Geometry: final body of the model. Coordinates: model frame, mm. A direction names the side the tool comes from. Round coordinates to 2 decimals unless told otherwise and drop trailing zeros. Write each loop counter-clockwise with the first axis right and the second up, starting at its lowest first coordinate (ties: lowest second). Pieces come first, ordered by that corner, then holes. Notation, with made-up numbers: (52.5, 58) -> (86.5, 58) arc R12 ccw to (86.5, 73) -> close; hole circle Ø9 at (70, 65.5). An arc over 180 degrees is marked (long way). One line per item, written item: value. Start each with the question number.
from build123d import *

# Parameters (mm, degrees)
AUFSATZ_LINEAR_AUSTRAGEN1_DEPTH = 120
SCHNITT_LINEAR_AUSTRAGEN1_DEPTH = 10
SKIZZE3_R                       = 3
SKIZZE3_R_2                     = 3.5
SCHNITT_LINEAR_AUSTRAGEN2_DEPTH = 60


with BuildPart() as part:
    # Skizze1 → Aufsatz-Linear austragen1 (new body)
    with BuildSketch(Plane.XY):
        with BuildLine():
            Line((0, 35), (0, 5))
            ThreePointArc((0, 5), (1.464466094, 1.464466094), (5, 0))
            Line((5, 0), (75, 0))
            ThreePointArc((75, 0), (78.535533906, 1.464466094), (80, 5))
            Line((80, 5), (80, 35))
            ThreePointArc((80, 35), (78.535533906, 38.535533906), (75, 40))
            Line((75, 40), (5, 40))
            ThreePointArc((5, 40), (1.464466094, 38.535533906), (0, 35))
        make_face()
        with BuildLine():
            Line((78, 5), (78, 35))
            ThreePointArc((78, 35), (77.121320344, 37.121320344), (75, 38))
            Line((75, 38), (5, 38))
            ThreePointArc((5, 38), (2.878679656, 37.121320344), (2, 35))
            Line((2, 35), (2, 5))
            ThreePointArc((2, 5), (2.878679656, 2.878679656), (5, 2))
            Line((5, 2), (75, 2))
            ThreePointArc((75, 2), (77.121320344, 2.878679656), (78, 5))
        make_face(mode=Mode.SUBTRACT)
    extrude(amount=AUFSATZ_LINEAR_AUSTRAGEN1_DEPTH)

    # Skizze2 → Schnitt-Linear austragen1 (cut)
    with BuildSketch(Plane.XZ):
        with BuildLine():
            Line((9, 120), (71, 120))
            Line((71, 120), (71, 75))
            ThreePointArc((71, 75), (69.535533906, 71.464466094), (66, 70))
            Line((66, 70), (14, 70))
            ThreePointArc((14, 70), (10.464466094, 71.464466094), (9, 75))
            Line((9, 75), (9, 120))
        make_face()
    extrude(amount=-SCHNITT_LINEAR_AUSTRAGEN1_DEPTH, mode=Mode.SUBTRACT)

    # Skizze3 → Schnitt-Linear austragen2 (cut)
    with BuildSketch(Plane(origin=(0, 40, 0), x_dir=(1, 0, 0), z_dir=(0, 1, 0))):
        with Locations(Location((60, -20, 0), (0, 0, 180))):
            Circle(SKIZZE3_R)
        with Locations(Location((20, -20, 0), (0, 0, 180))):
            Circle(SKIZZE3_R)
        with Locations(Location((60, -60, 0), (0, 0, 180))):
            Circle(SKIZZE3_R)
        with Locations(Location((20, -60, 0), (0, 0, 180))):
            Circle(SKIZZE3_R)
        with Locations(Location((63, -107, 0), (0, 0, 180))):
            Circle(SKIZZE3_R_2)
        with Locations(Location((17, -107, 0), (0, 0, 180))):
            Circle(SKIZZE3_R_2)
    extrude(amount=-SCHNITT_LINEAR_AUSTRAGEN2_DEPTH, mode=Mode.SUBTRACT)


solid = part.part
(1) Pull-direction query (Z, two-part tool) for faces 3 (the face through (11, 1, 71)), 4 (the face through (63, 1, 60)), 5 (the face through (2, 39, 59)); classes: pulls with the +Z half, pulls with the -Z half, needs draft (parallel to the pull), parting line crosses it, or undercut.
(2) Line query: probe 1 along Y at (x, z) = (58, 54.5); probe 2 along X at (y, z) = (32, 94); probe 3 along Y at (x, z) = (38.5, 74.5). Output: solid intervals per line, ascending.
(3) Section query C-C (y = 16). Output: boundary loops of the cut face in (x, z), and give its area (3 significant figures).
(4) Section query A-A (x = 28). Output: boundary loops of the cut face in (y, z).
(5) Section query D-D (z = 60). Count the separate pieces of the cut face and the enclosed holes in it, and give its area (3 significant figures).
(6) Pin query (flat end, axial travel): pin 1 (3 mm diameter, centred on x = 43.5, z = 79.5, fed in from -Y); pin 2 (3.5 mm diameter, centred on x = 60, z = 20, fed in from +Y); pin 3 (0.6 mm diameter, centred on y = 0.5, z = 93, fed in from +X); pin 4 (12 mm diameter, centred on x = 57, y = 6.5, fed in from +Z). Return the tip coordinate at first contact, or that it passes through.
(7) Set-up query: faces 1 (the face through (2, 20, 59)), 2 (the face through (17.759, 39.014, 103.583)). Return all of +Z, -Z, +X, -X, +Y, -Y with unobstructed straight access to the full face (end or side cutting, diameter ignored); none if empty.
(8) Section query B-B (z = 39). Output: boundary loops of the cut face in (x, y).
Results list:
1. face 3: pulls with the +Z half
1. face 4: undercut
1. face 5: needs draft
2. probe 1: y = 0 to 2, 38 to 40
2. probe 2: x = 0 to 2, 78 to 80
2. probe 3: y = 38 to 40
3. outline: (0, 0) -> (2, 0) -> (2, 120) -> (0, 120) -> close; (78, 0) -> (80, 0) -> (80, 120) -> (78, 120) -> close
3. area: 480 mm^2
4. outline: (0, 0) -> (2, 0) -> (2, 70) -> (0, 70) -> close; (38, 0) -> (40, 0) -> (40, 120) -> (38, 120) -> close
5. separate pieces: 4
5. enclosed holes: 0
5. area: 402 mm^2
6. pin 1: stops at y = 38
6. pin 2: passes through
6. pin 3: stops at x = 77.71
6. pin 4: stops at z = 70
7. face 1: +Z, -Z
7. face 2: +Y, -Y
8. outline: (0, 5) arc R5 ccw to (5, 0) -> (75, 0) arc R5 ccw to (80, 5) -> (80, 35) arc R5 ccw to (75, 40) -> (5, 40) arc R5 ccw to (0, 35) -> close; hole (2, 5) arc R3 ccw to (5, 2) -> (75, 2) arc R3 ccw to (78, 5) -> (78, 35) arc R3 ccw to (75, 38) -> (5, 38) arc R3 ccw to (2, 35) -> close
